Here's how the part is built. I have some questions about the finished solid (model axes, mm). A direction names the side the tool comes from. Coordinates: 2 decimals unless noted, no trailing zeros. Order: outer loops, then holes, each group sorted by start corner. A loop starts at its lowest first (then second) coordinate and runs counter-clockwise, first axis right, second up.
```python
from build123d import *

# Parameters (mm, degrees)
PATTERN_CIRCULAR_1_COUNT = 6
SKETCH_4_R               = 6
EXTRUDE_1_DEPTH          = 5
SKETCH_5_R               = 3
EXTRUDE_2_DEPTH          = 15
SKETCH_6_R               = 3.75
EXTRUDE_3_DEPTH          = 3
SKETCH_7_R               = 1
EXTRUDE_4_DEPTH          = 7
CUT_EXTRUDE_START        = -3
CUT_EXTRUDE_1_DEPTH      = 3
PATTERN_CIRCULAR_2_COUNT = 4
EXTRUDE_5_DEPTH          = 6.5
SKETCH_10_RX             = 1.5
SKETCH_10_RY             = 0.75
CUT_EXTRUDE_2_DEPTH      = 3
FILLET_1_R               = 0.5


with BuildPart() as part:
    # 草图1 → 旋转1 (revolve)
    with BuildSketch(Plane.XY, mode=Mode.PRIVATE) as revolve_1_sk:
        with BuildLine():
            Line((0, -0.5), (0, -44))
            Line((0, -44), (16.28, -44))
            ThreePointArc((16.28, -44), (16.421421356, -43.941421356), (16.48, -43.8))
            Line((16.48, -43.8), (16.48, -41))
            Line((16.48, -41), (16.5, -41))
            Line((16.5, -41), (16.5, -22))
            Line((16.5, -22), (18.5, -22))
            Line((18.5, -22), (18.5, 0))
            Line((18.5, 0), (12.7, 0))
            ThreePointArc((12.7, 0), (12.558578644, -0.058578644), (12.5, -0.2))
            Line((12.5, -0.2), (12.5, -0.5))
            Line((12.5, -0.5), (0, -0.5))
        make_face()
    revolve(revolve_1_sk.sketch.rotate(Axis((0, -0.5, 0), (0, -1, 0)), 90), axis=Axis((0, -0.5, 0), (0, -1, 0)))

    # 草图2 → M3 螺纹孔1 (revolve, cut)
    with BuildSketch(Plane(origin=(-15.5, 0, 0), x_dir=(0, 0, 1), z_dir=(1, 0, 0))):
        Polygon((0, 0), (0, 9.251075774), (1.25, 8.5), (1.25, 0), align=None)
    hole_wizard_m3_1 = revolve(axis=Axis((-15.5, 6.35, 0), (0, -1, 0)), mode=Mode.SUBTRACT)

    # 阵列(圆周)1: M3 螺纹孔1 ×6 about axis
    pattern_circular_1_axis = Axis((0, 0, 0), (0, 1, 0))
    for i in range(1, PATTERN_CIRCULAR_1_COUNT):
        add(hole_wizard_m3_1.rotate(pattern_circular_1_axis, i * 360 / PATTERN_CIRCULAR_1_COUNT), mode=Mode.SUBTRACT)

    # 草图4 → 凸台-拉伸1 (add)
    with BuildSketch(Plane(origin=(0, 0, 0), x_dir=(1, 0, 0), z_dir=(0, 1, 0))):
        with Locations(Location((0, 7, 0), (0, 0, 65.259733828))):
            Circle(SKETCH_4_R)
    extrude(amount=EXTRUDE_1_DEPTH)

    # 草图5 → 凸台-拉伸2 (add)
    with BuildSketch(Plane(origin=(0, 5, 0), x_dir=(1, 0, 0), z_dir=(0, 1, 0))):
        with Locations(Location((0, 7, 0), (0, 0, 180))):
            Circle(SKETCH_5_R)
    extrude(amount=EXTRUDE_2_DEPTH)

    # 草图6 → 凸台-拉伸3 (add)
    with BuildSketch(Plane.XZ.offset(44)):
        with Locations(Location((0, 0, 0), (0, 0, 90))):
            Circle(SKETCH_6_R)
    extrude(amount=EXTRUDE_3_DEPTH)

    # 草图7 → 凸台-拉伸4 (add)
    with BuildSketch(Plane.XZ.offset(47)):
        with Locations(Location((0, 0, 0), (0, 0, 270))):
            Circle(SKETCH_7_R)
    extrude(amount=EXTRUDE_4_DEPTH)

    # 草图8 → 切除-拉伸1 (cut)
    with BuildSketch(Plane.XZ.offset(44).offset(CUT_EXTRUDE_START)):
        with BuildLine():
            Line((-4.674811946, -15.803054555), (-3.814208524, -12.893811788))
            Line((-3.814208524, -12.893811788), (-1.200764091, -13.66691304))
            Line((-1.200764091, -13.66691304), (-1.996998191, -16.358557339))
            ThreePointArc((-1.996998191, -16.358557339), (-3.347448052, -16.136449161), (-4.674811946, -15.803054555))
        make_face()
    cut_extrude_1 = extrude(amount=CUT_EXTRUDE_1_DEPTH, mode=Mode.SUBTRACT)

    # 阵列(圆周)2: 切除-拉伸1 ×4 about axis
    pattern_circular_2_axis = Axis((0, 0, 0), (0, 1, 0))
    for i in range(1, PATTERN_CIRCULAR_2_COUNT):
        add(cut_extrude_1.rotate(pattern_circular_2_axis, i * 360 / PATTERN_CIRCULAR_2_COUNT), mode=Mode.SUBTRACT)

    # 草图9 → 凸台-拉伸5 (add)
    with BuildSketch(Plane.XZ.offset(44)):
        Polygon((-9.439875529, -7.318555185), (-7.318555185, -9.439875529), (-7.53068722, -9.652007563), (-9.652007563, -7.53068722), align=None)
        Polygon((7.53068722, 9.652007563), (7.318555185, 9.439875529), (9.439875529, 7.318555185), (9.652007563, 7.53068722), align=None)
    extrude(amount=EXTRUDE_5_DEPTH)

    # 草图10 → 切除-拉伸2 (cut)
    with BuildSketch(Plane(origin=(-8.591347391, 0, -8.591347391), x_dir=(-0.7071067811865307, 0, 0.7071067811865643), z_dir=(-0.7071067811865643, 0, -0.7071067811865307))):
        with Locations(Location((0, -48.5), (0, 0, -90))):
            Ellipse(SKETCH_10_RX, SKETCH_10_RY)
    cut_extrude_2 = extrude(amount=-CUT_EXTRUDE_2_DEPTH, mode=Mode.SUBTRACT)

    # 圆角1
    fillet_1_edges = [part.edges().sort_by_distance(p)[0] for p in [
        (7.424621202, -50.5, 9.545941546),
        (9.545941546, -50.5, 7.424621202),
        (-7.424621202, -50.5, -9.545941546),
        (-9.545941546, -50.5, -7.424621202),
    ]]
    fillet(fillet_1_edges, radius=FILLET_1_R)

    # 镜向5: 切除-拉伸2 across plane
    add(cut_extrude_2.mirror(Plane(origin=(0, 0, 0), x_dir=(-0.7071067811865388, 0, 0.7071067811865562), z_dir=(-0.7071067811865562, 0, -0.7071067811865388))), mode=Mode.SUBTRACT)


solid = part.part
```
Q1. Will these pins go through, and if not, where does the flat tip stop? pin 1 (12 mm diameter, centred on y = -35, z = -13.5, fed in from -X); pin 2 (3 mm diameter, centred on y = 11.5, z = -3.5, fed in from -X); pin 3 (1.8 mm diameter, centred on x = -8.5, z = -9, fed in from -Y).
Q2. I need wall thicknesses on L1, parallel to X at y = -3, z = 0; L2, parallel to Y at x = -4, z = -6.5; L3, parallel to Y at x = -2, z = 13. Which ranges of each line are inside material? Lowest first, please.
Q3. For faces 5 (the flat face through (-4.25, -42.48, -14.37)), 6 (the flat face through (14.37, -42.48, -4.25)), 7 (the flat face through (8.364, -46.482, 8.394)), 8 (the flat face through (0, 0, -7)), 9 (the cylindrical face through (-4.956, -31.367, 15.738)), which set-ups out of +Z, -Z, +X, -X, +Y, -Y let a thin tool reach every point of the face, with its end or its side?
Q4. We'd pull the mould along X, two halves only. Please class faces 1 (the flat face through (-8.576, -46.482, -8.606)), 2 (the flat face through (-4, -44, 0)), 3 (the cylindrical face through (-8.23, -4.19, 12.27)), 4 (the flat face through (-13.275, -42.479, 2.526)): pulls with the +X half, pulls with the -X half, needs draft (parallel to the pull), parting line crosses it, or undercut.
Q5. If we section it at A-A on y = -14: Write out the boundary of the cut face in (x, z).
Q6. If we section it at B-B on y = 11: Write out the boundary of the cut face in (x, z), then the cut area to 3 significant figures.
Reply:
1. pin 1: stops at x = -14.7
1. pin 2: stops at x = -2.24
1. pin 3: stops at y = -50.5
2. L1: x = -18.5 to -16.75, -14.25 to 14.25, 16.75 to 18.5
2. L2: y = -44 to -0.5, 0 to 5
2. L3: y = -44 to 0
3. face 5: -Z, -Y
3. face 6: +X, -Y
3. face 7: -Z, -X, -Y
3. face 8: none
3. face 9: -Y
4. face 1: pulls with the -X half
4. face 2: needs draft
4. face 3: undercut
4. face 4: undercut
5. outline: circle Ø37 at (0, 0)
6. outline: circle Ø6 at (0, -7)
6. area: 28.3 mm2
